Here's how the part is built. I have some questions about the finished solid (model axes, mm). Face numbers are marked on the shaded views. A direction names the side the tool comes from. Coordinates: 2 decimals unless noted, no trailing zeros. Use CSV: the item, a comma, the result in double quotes. Start each with the question number.
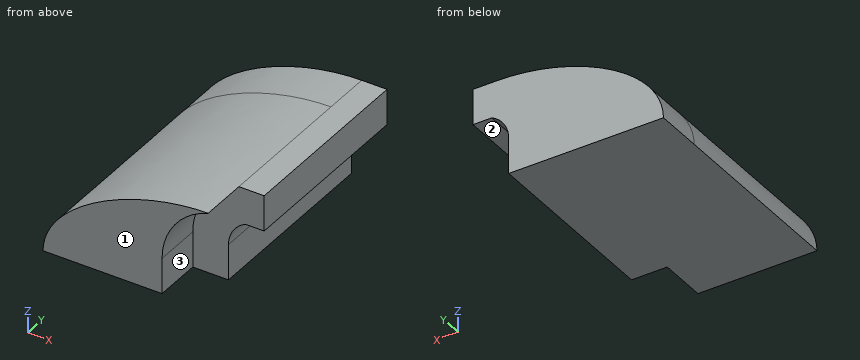
from build123d import *

# Parameters (mm, degrees)
F1_DEPTH = 25.4
F2_DEPTH = 101.6
F3_DEPTH = 101.6


with BuildPart() as f1:
    # F0 (on Front) → F1 (new body)
    with BuildSketch(Plane.XZ):
        with BuildLine():
            add(Edge.make_bspline(
                [(-41.275, 9.525), (-40.990595, 37.692979), (6.090595, 61.794065), (46.830385, 61.9252)],
                knots=[0, 0, 0, 0, 102.510194, 102.510194, 102.510194, 102.510194], degree=3))
            Line((-41.275, 9.525), (22.225, 9.525))
            Line((22.225, 9.525), (22.225, 28.559631))
            ThreePointArc((22.225, 28.559631), (29.041566, 49.288151), (46.830385, 61.9252))
        make_face()
    extrude(amount=F1_DEPTH)

    # F1_face (on face) → F2 (join)
    with BuildSketch(Plane(origin=(-1.16305, -25.4, 31.053726), x_dir=(1, 0, 0), z_dir=(0, -1, 0))):
        with BuildLine():
            add(Edge.make_bspline(
                [(-40.11195, -21.528726), (-39.827545, 6.639253), (7.253645, 30.740339), (47.993435, 30.871474)],
                knots=[0, 0, 0, 0, 102.510194, 102.510194, 102.510194, 102.510194], degree=3))
            Line((-40.11195, -21.528726), (23.38805, -21.528726))
            Line((23.38805, -21.528726), (23.38805, -2.494095))
            ThreePointArc((23.38805, -2.494095), (30.204616, 18.234425), (47.993435, 30.871474))
        make_face()
    extrude(amount=F2_DEPTH)

    # F0 (on Front) → F3 (join)
    with BuildSketch(Plane.XZ):
        with BuildLine():
            Line((22.225, 28.559631), (22.225, 9.525))
            Line((22.225, 9.525), (41.275, 9.525))
            Line((41.275, 9.525), (41.275, 28.559631))
            ThreePointArc((41.275, 28.559631), (43.716053, 37.018041), (50.288505, 42.8752))
            Line((50.288505, 42.8752), (60.325, 42.8752))
            Line((60.325, 42.8752), (60.325, 61.9252))
            Line((60.325, 61.9252), (46.830385, 61.9252))
            ThreePointArc((46.830385, 61.9252), (29.041566, 49.288151), (22.225, 28.559631))
        make_face()
    extrude(amount=F3_DEPTH)


solid = f1.part
Item 1: For pin 1 Ø11 at (x, y) = (56.5, -72) entering from -Z; pin 2 Ø19 at (x, z) = (48, 27.5) entering from -Y; pin 3 Ø15 at (y, z) = (-47, 18) entering from +X (3 decimals); pin 4 Ø1.5 at (x, z) = (-23.5, 41) entering from -Y, each with a flat end and sliding along its axis, tell me the tip position at first contact or that it passes through.
Item 2: For the marked faces 1, 2 and 3, which set-ups out of +Z, -Z, +X, -X, +Y, -Y let a thin tool reach every point of the face, with its end or its side?
Item 3: Please list where these lines run through material, in increasing order: line 1 along Y through (x, z) = (46, 51.5); line 2 along X through (y, z) = (-50, 52.5) (3 decimals); line 3 along Z through (x, y) = (-4, -45.5) (3 decimals). Write a range as from..to.
Here are the results:
1,pin 1,"z = 42.88"
1,pin 2,"y = -101.6"
1,pin 3,"x = 41.275"
1,pin 4,"through"
2,face 1,"+Z, -Z, +X, -X, -Y"
2,face 2,"-Z, +X, +Y, -Y"
2,face 3,"-Z, +X, -Y"
3,line 1,"-101.6..0"
3,line 2,"0.595..60.325"
3,line 3,"9.525..50.513"
